from build123d import *

# Parameters (mm, degrees)
CUT_EXTRUDE2_DEPTH = 2.5


with BuildPart() as part:
    # Sketch1 → Revolve1 (revolve)
    with BuildSketch(Plane(origin=(0, 0, 0), x_dir=(1, 0, 0), z_dir=(0, 1, 0)), mode=Mode.PRIVATE) as revolve1_sk:
        with BuildLine():
            Line((-2818.542001076, 1216.198145417), (-2818.542001076, 1223.198145417))
            Line((-2818.542001076, 1223.198145417), (-2821.042001076, 1223.198145417))
            Line((-2821.042001076, 1223.198145417), (-2821.042001076, 1214.285550771))
            Line((-2821.042001076, 1214.285550771), (-2820.196168753, 1214.285550771))
            Line((-2820.196168753, 1214.285550771), (-2820.196168753, 1211.285550771))
            Line((-2820.196168753, 1211.285550771), (-2818.542001076, 1211.285550771))
            Line((-2818.542001076, 1211.285550771), (-2816.542001076, 1211.285550771))
            Line((-2816.542001076, 1211.285550771), (-2816.542001076, 1198.198145417))
            Line((-2816.542001076, 1198.198145417), (-2813.542001076, 1198.198145417))
            Line((-2813.542001076, 1198.198145417), (-2813.542001076, 1205.198145417))
            Line((-2813.542001076, 1205.198145417), (-2814.542001076, 1205.198145417))
            ThreePointArc((-2814.542001076, 1205.198145417), (-2815.249107857, 1205.491038636), (-2815.542001076, 1206.198145417))
            Line((-2815.542001076, 1206.198145417), (-2815.542001076, 1216.198145417))
            Line((-2815.542001076, 1216.198145417), (-2818.542001076, 1216.198145417))
        make_face()
    revolve(revolve1_sk.sketch.rotate(Axis((-2823.542001076, 0, -1216.198145417), (0, 0, 1)), 180), axis=Axis((-2823.542001076, 0, -1216.198145417), (0, 0, 1)))

    # Sketch2 → Cut-Extrude2 (cut)
    with BuildSketch(Plane.XY.offset(-1211.285550771)):
        Polygon((-2819.327722789, 0), (-2821.434861933, 3.649672055), (-2825.649140219, 3.649672055), (-2827.756279362, 0), (-2825.649140219, -3.649672055), (-2821.434861933, -3.649672055), align=None)
    extrude(amount=-CUT_EXTRUDE2_DEPTH, mode=Mode.SUBTRACT)


solid = part.part
Input: part model. Units: mm. Frame: model coordinates. A direction names the side the tool comes from. Coordinates: 2 decimals unless noted, no trailing zeros. Loops run counter-clockwise (first coordinate to the right, second up) from the corner with the lowest first, then second, coordinate; pieces in that order, holes last. Notation, with made-up numbers: (14, 89.5) - (56, 89.5) arc R15 cw to (56, 116.5) - close; hole circle Ø1 at (23.5, 26.25). An arc over 180 degrees is marked (long way). Answer in a Markdown table with one row per item. Add a question column.
Item 1: Section query B-B on z = -1218.5. Return the cut outline in (x, y), then the cut area to 3 significant figures.
Item 2: Line query: line 1 along Z through (x, y) = (-2826.25, 3.5); line 2 along Z through (x, y) = (-2817, 1.5); line 3 along Y through (x, z) = (-2822, -1211.75). Output: solid intervals per line, ascending. Write a range as [from, to].
Item 3: Contact query for flat-ended pins moving along their axis: P1, Ø0.8, axis at x = -2822.5, z = -1212, coming from the +Y side; P2, Ø1.5, axis at y = 6, z = -1201, coming from the +X side; P3, Ø1, axis at x = -2821, z = -1202, coming from the +Y side. Output: stop coordinate, or through.
Item 4: Mould query, pull axis X, two halves, no side actions, for faces 4 (the cylindrical face through (-2832.78, 3.83, -1201.75)), 5 (the flat face through (-2821, -7, -1198.198)), 6 (the flat face through (-2824, -3.65, -1213)). Classes: released by +X, released by -X, zero draft, split by the parting line, or undercut.
Item 5: Access query for faces 1 (the flat face through (-2826.717, -1.799, -1212.518)), 2 (the cylindrical face through (-2828.31, -1.5, -1219.75)), 3 (the flat face through (-2821, 1, -1223.198)). Directions: +Z, -Z, +X, -X, +Y, -Y. A direction counts if a zero-diameter tool reaches every point of the face in a straight line with its end or side. Return the directions, or none.
Item 6: Section query A-A on z = -1208. Return the cut outline in (x, y).
Recorded:
| question | item | result |
|---|---|---|
| 1 | outline | circle Ø10 at (-2823.54, 0); hole circle Ø5 at (-2823.54, 0) |
| 1 | area | 58.9 mm^2 |
| 2 | line 1 | [-1223.2, -1211.29] |
| 2 | line 2 | [-1216.2, -1211.29] |
| 2 | line 3 | [-7.85, -3.65], [3.65, 7.85] |
| 3 | P1 | y = 7.97 |
| 3 | P2 | x = -2815.03 |
| 3 | P3 | y = 9.79 |
| 4 | face 4 | split by the parting line |
| 4 | face 5 | zero draft |
| 4 | face 6 | undercut |
| 5 | face 1 | +Z |
| 5 | face 2 | -Z |
| 5 | face 3 | -Z, +X, -X, +Y, -Y |
| 6 | outline | circle Ø16 at (-2823.54, 0); hole circle Ø14 at (-2823.54, 0) |
